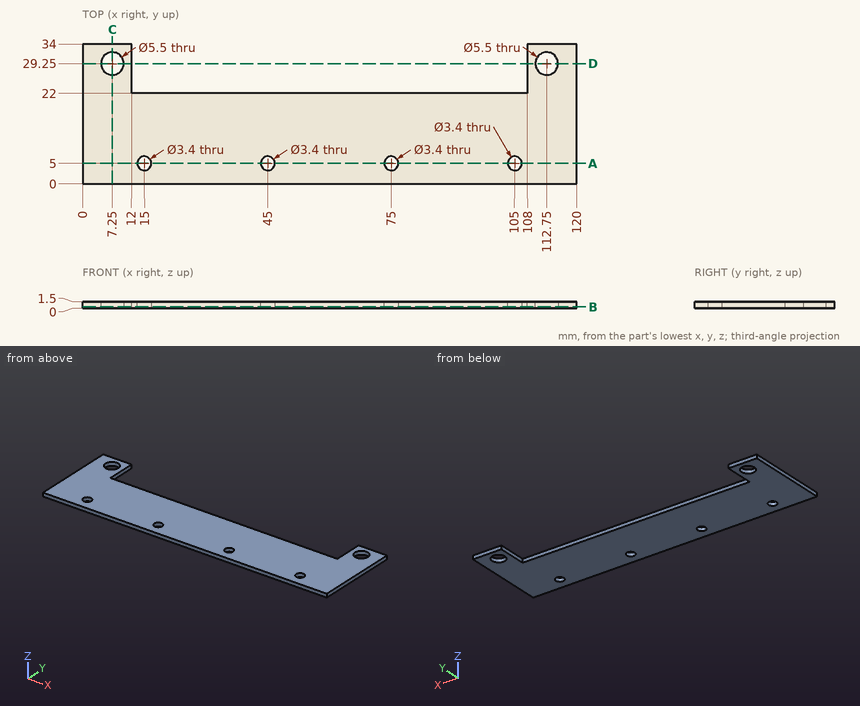
Part print with two shaded views. Sizes in mm from the minimum x, y, z corner. Round coordinates to 2 decimals unless told otherwise and drop trailing zeros. Order: outer loops, then holes, each group sorted by start corner. A loop starts at its lowest first (then second) coordinate and runs counter-clockwise, first axis right, second up. Notation, with made-up numbers: M 71,87 L 120,87 A32 cw 120,113 Z; hole C -5,-24 d11. An arc over 180 degrees is marked long. Answer in a Markdown table with one row per item. Add a question column.
Q1. Wall check: L1, parallel to X at y = 27, z = 0.8; L2, parallel to Y at x = 112.75, z = 0.45; L3, parallel to Y at x = 105, z = 0.4. Give the ranges that are in metal, low to high. Write a range as from..to.
Q2. Cut at D-D on y = 29.25. Give the cut face in (x, z), and give its area (3 significant figures).
Q3. Pin check, flat tip, straight feed: pin 1 (1.5 mm diameter, centred on x = 66.5, y = 24.5, fed in from +Z). Stop position of the tip, or through.
Q4. Cut at A-A on y = 5. Give the cut face in (x, z).
Q5. Cut at B-B on z = 0.3. Give the cut face in (x, y).
Q6. Cut at C-C on x = 7.25. Give the cut face in (y, z), and give its area (4 significant figures).
Established:
| question | item | result |
|---|---|---|
| 1 | L1 | x = 0..5.67, 8.83..12, 108..111.17, 114.33..120 |
| 1 | L2 | y = 0..26.5, 32..34 |
| 1 | L3 | y = 0..3.3, 6.7..22 |
| 2 | outline | M 0,0 L 4.5,0 L 4.5,1.5 L 0,1.5 Z; M 10,0 L 12,0 L 12,1.5 L 10,1.5 Z; M 108,0 L 110,0 L 110,1.5 L 108,1.5 Z; M 115.5,0 L 120,0 L 120,1.5 L 115.5,1.5 Z |
| 2 | area | 19.5 mm2 |
| 3 | pin 1 | passes through |
| 4 | outline | M 0,0 L 13.3,0 L 13.3,1.5 L 0,1.5 Z; M 16.7,0 L 43.3,0 L 43.3,1.5 L 16.7,1.5 Z; M 46.7,0 L 73.3,0 L 73.3,1.5 L 46.7,1.5 Z; M 76.7,0 L 103.3,0 L 103.3,1.5 L 76.7,1.5 Z; M 106.7,0 L 120,0 L 120,1.5 L 106.7,1.5 Z |
| 5 | outline | M 0,0 L 120,0 L 120,34 L 108,34 L 108,22 L 12,22 L 12,34 L 0,34 Z; hole C 7.25,29.25 d5.5; hole C 15,5 d3.4; hole C 45,5 d3.4; hole C 75,5 d3.4; hole C 105,5 d3.4; hole C 112.75,29.25 d5.5 |
| 6 | outline | M 0,0 L 26.5,0 L 26.5,1.5 L 0,1.5 Z; M 32,0 L 34,0 L 34,1.5 L 32,1.5 Z |
| 6 | area | 42.75 mm2 |
